The listing builds one solid part. Answer for the finished solid, in the listing's coordinates (mm). Face numbers are marked on the shaded views. A direction names the side the tool comes from. Round coordinates to 2 decimals unless told otherwise and drop trailing zeros. Loops run counter-clockwise (first coordinate to the right, second up) from the corner with the lowest first, then second, coordinate; pieces in that order, holes last. Notation, with made-up numbers: (43, 23) - (47, 23) arc R31 ccw to (47, 51) - close; hole circle Ø1 at (-35.75, 53.5). An arc over 180 degrees is marked (long way). One line per question, with ' | ' between items. Start each with the question number.
from build123d import *

# Parameters (mm, degrees)
SKETCH1_W           = 38.1
SKETCH1_H           = 28.448
BOSS_EXTRUDE1_DEPTH = 12.7
CUT_EXTRUDE2_REACH  = 14.7
FILLET1_R           = 0.254


with BuildPart() as part:
    # Sketch1 → Boss-Extrude1 (new body)
    with BuildSketch(Plane.XY):
        with Locations((19.05, 14.224)):
            Rectangle(SKETCH1_W, SKETCH1_H)
    extrude(amount=-BOSS_EXTRUDE1_DEPTH)

    # Sketch3 → Cut-Extrude2 (cut, up to next)
    with BuildSketch(Plane.XY, mode=Mode.PRIVATE) as cut_extrude2_sk1:
        with BuildLine():
            Line((16.66875, 28.448), (16.66875, 23.446541593))
            ThreePointArc((16.66875, 23.446541593), (19.05, 4.699), (21.43125, 23.446541593))
            Line((21.43125, 23.446541593), (21.43125, 28.448))
            Line((21.43125, 28.448), (16.66875, 28.448))
        make_face()
    cut_extrude2_tool1 = extrude(cut_extrude2_sk1.sketch, amount=-CUT_EXTRUDE2_REACH, mode=Mode.PRIVATE) & part.part
    add(cut_extrude2_tool1.solids().sort_by_distance((19.05, 15.101748, 0))[0], mode=Mode.SUBTRACT)

    # Fillet1
    fillet1_edges = [part.edges().sort_by_distance(p)[0] for p in [
        (38.1, 14.224, -12.7),
        (8.334375, 28.448, 0),
        (8.334375, 28.448, -12.7),
        (29.765625, 28.448, -12.7),
        (21.43125, 23.446541593, -6.35),
        (16.66875, 23.446541593, -6.35),
        (16.66875, 28.448, -6.35),
        (21.43125, 25.947270797, -12.7),
        (21.43125, 28.448, -6.35),
        (21.43125, 25.947270797, 0),
        (19.05, 4.699, 0),
        (16.66875, 25.947270797, 0),
        (19.05, 4.699, -12.7),
        (16.66875, 25.947270797, -12.7),
        (0, 14.224, -12.7),
        (29.765625, 28.448, 0),
        (38.1, 14.224, 0),
        (19.05, 0, 0),
        (0, 14.224, 0),
        (0, 28.448, -6.35),
        (38.1, 28.448, -6.35),
        (38.1, 0, -6.35),
        (0, 0, -6.35),
        (19.05, 0, -12.7),
    ]]
    fillet(fillet1_edges, radius=FILLET1_R)


solid = part.part
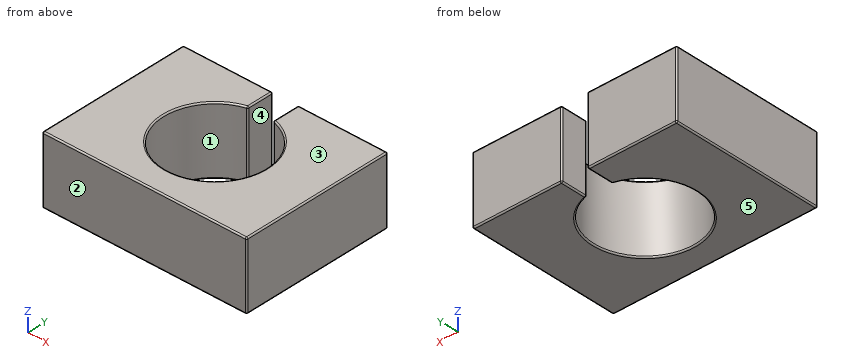
(1) Consider L1, parallel to X at y = 25, z = -6.75; L2, parallel to X at y = 14.5, z = -2; L3, parallel to Y at x = 19.05, z = -8. Determine where each line is inside the solid, lowest interval first.
(2) A tool of negligible diameter and unlimited length cuts with its end or side. For the marked faces 4 and 5, from which of +Z, -Z, +X, -X, +Y, -Y can it reach the whole face along a straight path? Write none if from no direction.
(3) This flat-tipped pin is pushed along its axis until it touches: P1, Ø3, axis at x = 17, y = 21.5, coming from the -Z side. Where does it stop, or does it pass through?
(4) Find section B-B on x = 19.05. Write down the section's boundary in (y, z) (3 decimals), plus the area to 3 significant figures.
(5) Determine the mould class of the marked faces 1, 2 and 3 for opening direction Y: pulls with the +Y half, pulls with the -Y half, needs draft (parallel to the pull), parting line crosses it, or undercut.
(6) Find section A-A on z = -10.5. Write down the section's boundary in (x, y) (3 decimals), plus the area to 3 significant figures.
Answer below:
1) L1: 0 to 16.67, 21.43 to 38.1 | L2: 0 to 9.53, 28.57 to 38.1 | L3: 0 to 4.7
2) face 4: +Z, -Z, +Y | face 5: -Z, +X, -X, +Y, -Y
3) P1: through
4) outline: (0, -12.446) arc R0.254 ccw to (0.254, -12.7) - (4.445, -12.7) arc R0.254 ccw to (4.699, -12.446) - (4.699, -0.254) arc R0.254 ccw to (4.445, 0) - (0.254, 0) arc R0.254 ccw to (0, -0.254) - close | area: 59.6 mm2
5) face 1: undercut | face 2: pulls with the -Y half | face 3: needs draft
6) outline: (0, 0.254) arc R0.254 ccw to (0.254, 0) - (37.846, 0) arc R0.254 ccw to (38.1, 0.254) - (38.1, 28.194) arc R0.254 ccw to (37.846, 28.448) - (21.685, 28.448) arc R0.254 ccw to (21.431, 28.194) - (21.431, 23.641) arc R0.254 ccw to (21.617, 23.397) arc R9.525 cw (long way) to (16.483, 23.397) arc R0.254 ccw to (16.669, 23.641) - (16.669, 28.194) arc R0.254 ccw to (16.415, 28.448) - (0.254, 28.448) arc R0.254 ccw to (0, 28.194) - close | area: 776 mm2
